from build123d import *

# Parameters (mm, degrees)
SKETCH2_W           = 65
SKETCH2_H           = 65
BOSS_EXTRUDE1_DEPTH = 65
SKETCH3_W           = 57
SKETCH3_H           = 57
CUT_EXTRUDE1_DEPTH  = 57
CUT_EXTRUDE2_DEPTH  = 9
CUT_EXTRUDE3_DEPTH  = 9
SKETCH8_R           = 12.5
CUT_EXTRUDE4_DEPTH  = 66


with BuildPart() as part:
    # Sketch2 → Boss-Extrude1 (new body)
    with BuildSketch(Plane.XY):
        Rectangle(SKETCH2_W, SKETCH2_H)
    extrude(amount=BOSS_EXTRUDE1_DEPTH)

    # Sketch3 → Cut-Extrude1 (cut)
    with BuildSketch(Plane.XY.offset(65)):
        with Locations((4, -4)):
            Rectangle(SKETCH3_W, SKETCH3_H)
    extrude(amount=-CUT_EXTRUDE1_DEPTH, mode=Mode.SUBTRACT)

    # Sketch5 → Cut-Extrude2 (cut, through all)
    with BuildSketch(Plane(origin=(-24.5, 0, 0), x_dir=(0, 0, -1), z_dir=(1, 0, 0))):
        Polygon((-65, -32.5), (-65, 24.5), (-8, -32.5), align=None)
    extrude(amount=-CUT_EXTRUDE2_DEPTH, mode=Mode.SUBTRACT)

    # Sketch7 → Cut-Extrude3 (cut, through all)
    with BuildSketch(Plane(origin=(0, 24.5, 0), x_dir=(-1, 0, 0), z_dir=(0, -1, 0))):
        Polygon((-32.5, -65), (-5.5, -65), (-32.5, -38), align=None)
    extrude(amount=-CUT_EXTRUDE3_DEPTH, mode=Mode.SUBTRACT)

    # Sketch8 → Cut-Extrude4 (cut, through all)
    with BuildSketch(Plane(origin=(0, 0, 0), x_dir=(-1, 0, 0), z_dir=(0, 0, -1))):
        with Locations((-2.5, -2.5)):
            Circle(SKETCH8_R)
    extrude(amount=-CUT_EXTRUDE4_DEPTH, mode=Mode.SUBTRACT)


solid = part.part
The model under review builds one solid part; all positions refer to its coordinate system, in mm. A direction names the side the tool comes from. Coordinates: 2 decimals unless noted, no trailing zeros. Order: outer loops, then holes, each group sorted by start corner. A loop starts at its lowest first (then second) coordinate and runs counter-clockwise, first axis right, second up. Notation, with made-up numbers: (-33.75, -19) -> (-21.75, -19) arc R10 ccw to (-21.75, -7) -> close; hole circle Ø1 at (45, -2.75). An arc over 180 degrees is marked (long way). Answer in a Markdown table with one row per item.
(1) Insertion check: pin 1 (2 mm diameter, centred on x = -25, y = 6.5, fed in from +Z); pin 2 (6 mm diameter, centred on y = 25, z = 46, fed in from +X); pin 3 (6 mm diameter, centred on x = 24, y = 8.5, fed in from +Z). Each pin has a flat end and moves straight along its axis. Give the tip position at first contact, or say it passes through.
Answers:
| item | result |
|---|---|
| pin 1 | z = 48 |
| pin 2 | x = 27.5 |
| pin 3 | z = 8 |
(2) Consider section C-C (z = 27). Write out the cut boundary in (x, y).
Answers:
| item | result |
|---|---|
| outline | (-32.5, -13.5) -> (-24.5, -13.5) -> (-24.5, 24.5) -> (32.5, 24.5) -> (32.5, 32.5) -> (-32.5, 32.5) -> close |
(3) Consider section A-A (x = 2.5). Write out the cut boundary in (y, z), plus the area to 3 significant figures.
Answers:
| item | result |
|---|---|
| outline | (-32.5, 0) -> (-15, 0) -> (-15, 8) -> (-32.5, 8) -> close; (10, 0) -> (32.5, 0) -> (32.5, 65) -> (24.5, 65) -> (24.5, 8) -> (10, 8) -> close |
| area | 776 mm² |
(4) Consider section B-B (y = -2.5). Write out the cut boundary in (x, z), plus the area to 3 significant figures.
Answers:
| item | result |
|---|---|
| outline | (-32.5, 0) -> (-10, 0) -> (-10, 8) -> (-24.5, 8) -> (-24.5, 38) -> (-32.5, 38) -> close; (15, 0) -> (32.5, 0) -> (32.5, 8) -> (15, 8) -> close |
| area | 560 mm² |
(5) Wall thickness on line 1 along Y through (x, z) = (2, 2); line 2 along X through (y, z) = (-2, 5); line 3 along Z through (x, y) = (9, -25): over which ranges is each line inside the solid? List them lowest first.
Answers:
| item | result |
|---|---|
| line 1 | -32.5 to -14.99, 9.99 to 32.5 |
| line 2 | -32.5 to -9.99, 14.99 to 32.5 |
| line 3 | 0 to 8 |
(6) Consider section D-D (y = 25.5). Write out the cut boundary in (x, z), plus the area to 3 significant figures.
Answers:
| item | result |
|---|---|
| outline | (-32.5, 0) -> (32.5, 0) -> (32.5, 38) -> (5.5, 65) -> (-32.5, 65) -> close |
| area | 3,860 mm² |
(7) Machinability: for faces 1 (the flat face through (16, -4, 8)), 2 (the flat face through (32.5, 4.7, 7.7)), which of the approach directions +Z, -Z, +X, -X, +Y, -Y give a long, thin tool a straight path to every point of the face, cutting with its end or side? Answer none if there is none.
Answers:
| item | result |
|---|---|
| face 1 | +Z, +X, -Y |
| face 2 | +Z, -Z, +X, +Y, -Y |
